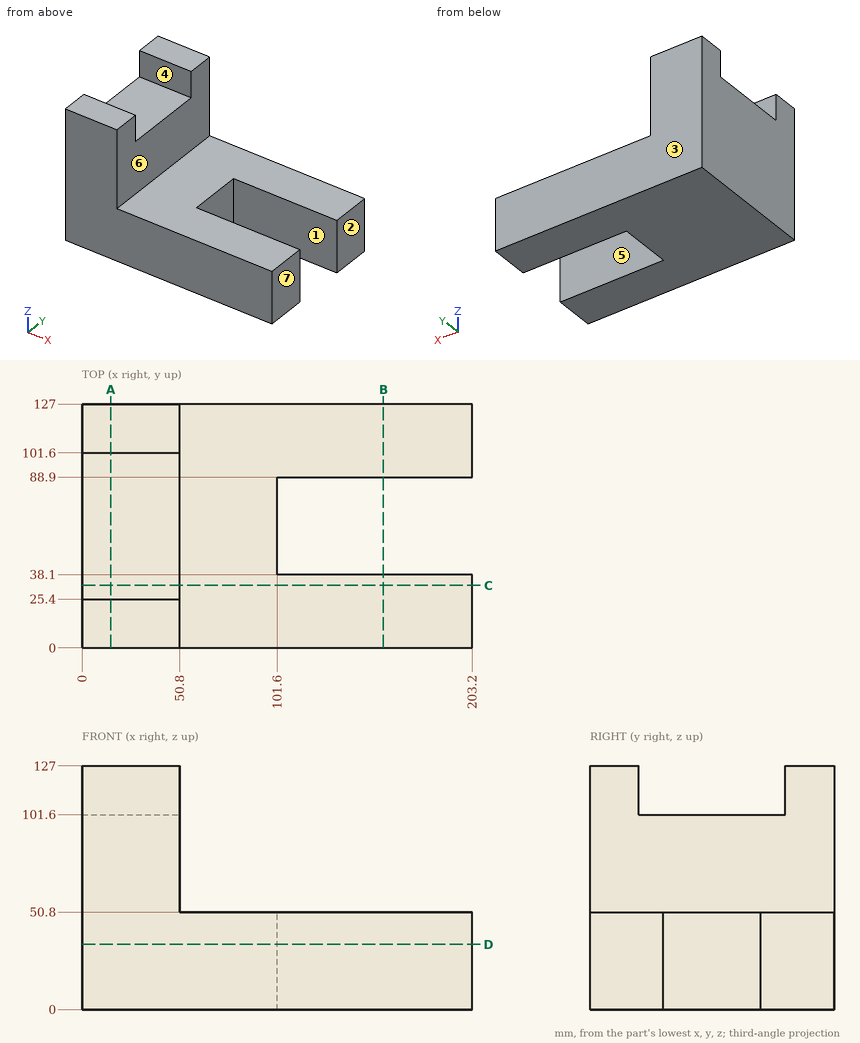
Print and shaded views of the part. All mm, measured from the part's lowest x, y and z. A direction names the side the tool comes from. Give positions to 0.01 mm unless a question says otherwise; leave off trailing zeros. Write each loop counter-clockwise with the first axis right and the second up, starting at its lowest first coordinate (ties: lowest second). Pieces come first, ordered by that corner, then holes. Notation, with made-up numbers: (69, 25) -> (93, 25) arc R19 cw to (93, 55) -> close; hole circle Ø2 at (-27.75, 70.5). An arc over 180 degrees is marked (long way). Use CSV: the item, a comma, the result in double quotes. Start each with the question number.
1) Cut at D-D on z = 34. List the corners of the cut face in (x, y), plus the area to 3 significant figures.
2) Cut at A-A on x = 15. List the corners of the cut face in (y, z), plus the area to 3 significant figures.
3) Two-plate mould, pull along Y, no slides. Class the marked faces 1, 2 and 3: released by +Y, released by -Y, zero draft, split by the parting line, or undercut.
4) Cut at C-C on y = 32.5. List the corners of the cut face in (x, z).
5) Drill centre lines: L1, parallel to Y at x = 151, z = 25.5; L2, parallel to Y at x = 13.5, z = 112; L3, parallel to Z at x = 43.5, y = 98.5. Where is each one in solid material? Low to high.
6) Pin check, flat tip, straight feed: P1, Ø23, axis at y = 78.5, z = 74.5, coming from the +X side. Stop position of the tip, or through.
7) Tool access for the marked faces 4, 5, 6 and 7: list every direction of +Z, -Z, +X, -X, +Y, -Y with a clear straight run to the whole face (end or side of a thin tool).
8) Cut at B-B on x = 157. List the corners of the cut face in (y, z), plus the area to 3 significant figures.
Final values:
1,outline,"(0, 0) -> (203.2, 0) -> (203.2, 38.1) -> (101.6, 38.1) -> (101.6, 88.9) -> (203.2, 88.9) -> (203.2, 127) -> (0, 127) -> close"
1,area,"20,600 mm2"
2,outline,"(0, 0) -> (127, 0) -> (127, 127) -> (101.6, 127) -> (101.6, 101.6) -> (25.4, 101.6) -> (25.4, 127) -> (0, 127) -> close"
2,area,"14,200 mm2"
3,face 1,"undercut"
3,face 2,"zero draft"
3,face 3,"released by +Y"
4,outline,"(0, 0) -> (203.2, 0) -> (203.2, 50.8) -> (50.8, 50.8) -> (50.8, 101.6) -> (0, 101.6) -> close"
5,L1,"y = 0 to 38.1, 88.9 to 127"
5,L2,"y = 0 to 25.4, 101.6 to 127"
5,L3,"z = 0 to 101.6"
6,P1,"stops at x = 50.8"
7,face 4,"+Z, +X, -X"
7,face 5,"+Z, -Z, +X"
7,face 6,"+Z, +X, +Y, -Y"
7,face 7,"+Z, -Z, +X, +Y, -Y"
8,outline,"(0, 0) -> (38.1, 0) -> (38.1, 50.8) -> (0, 50.8) -> close; (88.9, 0) -> (127, 0) -> (127, 50.8) -> (88.9, 50.8) -> close"
8,area,"3,870 mm2"
